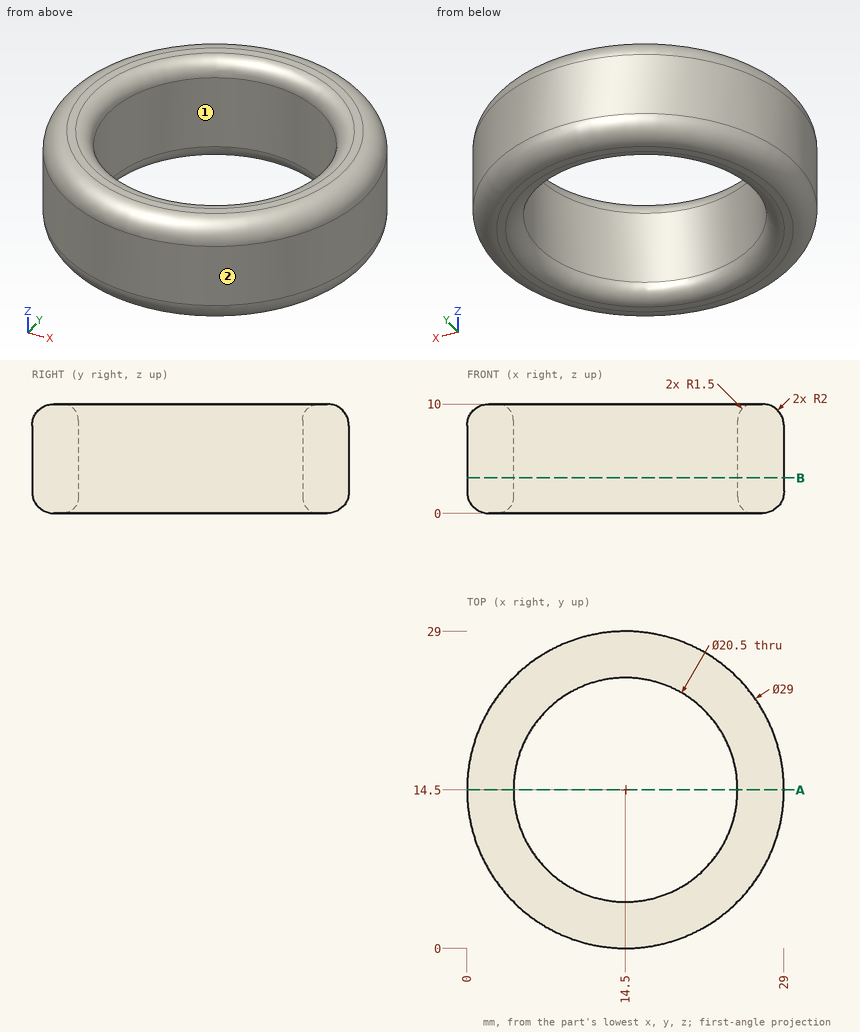
Here's the drawing with two shaded views (mm, measured from the low corner). I have some questions. Round coordinates to 2 decimals unless told otherwise and drop trailing zeros. Loops run counter-clockwise (first coordinate to the right, second up) from the corner with the lowest first, then second, coordinate; pieces in that order, holes last. Notation, with made-up numbers: (6.5, -22.5) - (64.5, -22.5) arc R21 ccw to (64.5, -9.5) - close; hole circle Ø2 at (-33, -18). An arc over 180 degrees is marked (long way). Use CSV: the item, a comma, the result in double quotes. Start each with the question number.
1) We'd pull the mould along Y, two halves only. Please class the marked faces 1 and 2: released by +Y, released by -Y, zero draft, split by the parting line, or undercut.
2) For pin 1 Ø2 at (y, z) = (17.5, 4) entering from +X; pin 2 Ø4 at (y, z) = (10, 9) entering from -X; pin 3 Ø5 at (x, z) = (20.5, 1.5) entering from -Y, each with a flat end and sliding along its axis, tell me the tip position at first contact or that it passes through.
3) If we section it at A-A on y = 14.5: Write out the boundary of the cut face in (x, z).
4) Please list where these lines run through material, in increasing order: probe 1 along Y at (x, z) = (14.5, 3); probe 2 along Y at (x, z) = (21, 3.75); probe 3 along X at (y, z) = (5.75, 6). Write a range as [from, to].
5) If we section it at B-B on z = 3.25: Write out the boundary of the cut face in (x, y), plus the area to 3 significant figures.
Geometry results:
1,face 1,"undercut"
1,face 2,"split by the parting line"
2,pin 1,"stops at x = 28.86"
2,pin 2,"stops at x = 0.26"
2,pin 3,"stops at y = 0.44"
3,outline,"(0, 2) arc R2 ccw to (2, 0) - (2.75, 0) arc R1.5 ccw to (4.25, 1.5) - (4.25, 8.5) arc R1.5 ccw to (2.75, 10) - (2, 10) arc R2 ccw to (0, 8) - close; (24.75, 1.5) arc R1.5 ccw to (26.25, 0) - (27, 0) arc R2 ccw to (29, 2) - (29, 8) arc R2 ccw to (27, 10) - (26.25, 10) arc R1.5 ccw to (24.75, 8.5) - close"
4,probe 1,"y = [0, 4.25], [24.75, 29]"
4,probe 2,"y = [1.54, 6.57], [22.43, 27.46]"
4,probe 3,"x = [2.94, 9.16], [19.84, 26.06]"
5,outline,"circle Ø29 at (14.5, 14.5); hole circle Ø20.5 at (14.5, 14.5)"
5,area,"330 mm2"
